Source: CAD feature listing. Evaluate the final solid. Frame: model axes, mm. Face numbers are marked on the shaded views. A direction names the side the tool comes from. Give positions to 0.01 mm unless a question says otherwise; leave off trailing zeros. Loops run counter-clockwise (first coordinate to the right, second up) from the corner with the lowest first, then second, coordinate; pieces in that order, holes last. Notation, with made-up numbers: M 17,53 L 63,53 A18 ccw 63,85 Z; hole C 34,39 d4. An arc over 180 degrees is marked long. Write item = value, one per line.
from build123d import *

# Parameters (mm, degrees)
SKETCH1_R           = 8.9
SKETCH1_R_2         = 4
BOSS_EXTRUDE1_DEPTH = 2
CUT_EXTRUDE1_DEPTH  = 2
SKETCH3_R           = 5
SKETCH3_R_2         = 4
BOSS_EXTRUDE2_DEPTH = 5
SKETCH4_R           = 4.075
CUT_EXTRUDE2_DEPTH  = 15
SKETCH6_R           = 1
CUT_EXTRUDE3_DEPTH  = 15


with BuildPart() as part:
    # Sketch1 → Boss-Extrude1 (new body)
    with BuildSketch(Plane(origin=(0, 0, 0), x_dir=(1, 0, 0), z_dir=(0, 1, 0))):
        Circle(SKETCH1_R)
        Circle(SKETCH1_R_2, mode=Mode.SUBTRACT)
    extrude(amount=BOSS_EXTRUDE1_DEPTH)

    # Sketch2 → Cut-Extrude1 (cut)
    with BuildSketch(Plane(origin=(0, 2, 0), x_dir=(1, 0, 0), z_dir=(0, 1, 0))):
        Polygon((0, 0), (0, -10.52604124), (-0.355401251, -10.177360244), align=None)
    extrude(amount=-CUT_EXTRUDE1_DEPTH, mode=Mode.SUBTRACT)

    # Sketch3 → Boss-Extrude2 (add)
    with BuildSketch(Plane(origin=(0, 2, 0), x_dir=(1, 0, 0), z_dir=(0, 1, 0))):
        Circle(SKETCH3_R)
        Circle(SKETCH3_R_2, mode=Mode.SUBTRACT)
    extrude(amount=-BOSS_EXTRUDE2_DEPTH)

    # Sketch4 → Cut-Extrude2 (cut)
    with BuildSketch(Plane(origin=(0, 2, 0), x_dir=(1, 0, 0), z_dir=(0, 1, 0))):
        Circle(SKETCH4_R)
    extrude(amount=-CUT_EXTRUDE2_DEPTH, mode=Mode.SUBTRACT)

    # Sketch6 → Cut-Extrude3 (cut)
    with BuildSketch(Plane.XY):
        with Locations((0, -1.5)):
            Circle(SKETCH6_R)
    extrude(amount=-CUT_EXTRUDE3_DEPTH, mode=Mode.SUBTRACT)


solid = part.part
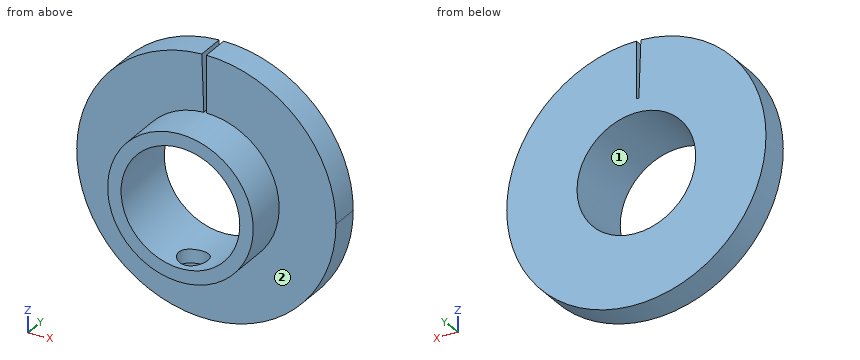
1. Cut plane D-D, the plane z = -1. Return the cut outline in (x, y).
Derived:
outline = M -8.84,0 L -4.9,0 L -4.9,-3 L -3.95,-3 L -3.95,2 L -8.84,2 Z; M 3.95,-3 L 4.9,-3 L 4.9,0 L 8.84,0 L 8.84,2 L 3.95,2 Z
2. Material intervals for probe 1 along X at (y, z) = (-1, 0) (3 decimals); probe 2 along X at (y, z) = (0.7, 0) (3 decimals); probe 3 along Y at (x, z) = (0, -4.35), sorted ascending. Write a range as from..to.
Derived:
probe_1 = -5..-4.075, 4.075..5
probe_2 = -8.9..-4.075, 4.075..8.9
probe_3 = -3..-2.5, -0.5..2
3. First-contact query: pin 1 Ø1.6 at (x, y) = (0, -1.5) entering from +Z; pin 2 Ø3 at (x, y) = (3.5, 0.5) entering from -Z; pin 3 Ø2 at (x, y) = (-3.5, -2.5) entering from +Z. Flat tips, straight axial feed; report the tip coordinate or a pass-through.
Derived:
pin_1 = 5
pin_2 = -8.67
pin_3 = 4.33
4. Reachability of the marked faces 1 and 2 from +Z, -Z, +X, -X, +Y, -Y: full face, straight path, thin tool, end or side. Return the list, or none.
Derived:
face_1 = +Y, -Y
face_2 = -Y
5. Cut plane C-C, the plane x = -4.75. Return the cut outline in (y, z), then the cut area to 3 significant figures.
Derived:
outline = M -3,-1.56 L 0,-1.56 L 0,-7.53 L 2,-7.53 L 2,7.53 L 0,7.53 L 0,1.56 L -3,1.56 Z
area = 39.5 mm²
6. Cut plane A-A, the plane z = 6.5. Return the cut outline in (x, y).
Derived:
outline = M -6.08,0 L -0.23,0 L -0.23,2 L -6.08,2 Z; M 0,0 L 6.08,0 L 6.08,2 L 0,2 Z
